Model file for the job. Use its own axes, mm. A direction names the side the tool comes from. Round coordinates to 2 decimals unless told otherwise and drop trailing zeros. Order: outer loops, then holes, each group sorted by start corner. A loop starts at its lowest first (then second) coordinate and runs counter-clockwise, first axis right, second up. Notation, with made-up numbers: (8, 24) - (64, 24) arc R25 ccw to (64, 43) - close; hole circle Ø4 at (54, -36.5). An arc over 180 degrees is marked (long way). Write item = value, one per line.
```python
from build123d import *

# Parameters (mm, degrees)
R_VOL_MINCE1_OUTLINE_W = 0.5
R_VOL_MINCE1_OUTLINE_H = 1
CONG_2_R               = 8
CONG_3_R               = 8


# Read off the part's stored shape, not the designer's step: Révol.-Mince1
with BuildPart() as part:
    # Révol.-Mince1 outline → Révol.-Mince1 (revolve)
    with BuildSketch(Plane.XY):
        Polygon((2.5, 5), (2.5, 0), (7, 0), (7, 23.528490035), (26.111064682, 23.528490035), (29, 0), (34.646665968, 0), (34.646665968, 3), (30.646665968, 3), (27.880515211, 25.528490035), (5, 25.528490035), (5, 5), align=None)
        with Locations((4.75, 2.5)):
            Rectangle(R_VOL_MINCE1_OUTLINE_W, R_VOL_MINCE1_OUTLINE_H, mode=Mode.SUBTRACT)
    revolve(axis=Axis((0, 0, 0), (0, 1, 0)))

    # Congé2
    cong_2_edges = [part.edges().sort_by_distance(p)[0] for p in [
        (-26.111064682, 23.528490035, 0),
    ]]
    fillet(cong_2_edges, radius=CONG_2_R)

    # Congé3
    cong_3_edges = [part.edges().sort_by_distance(p)[0] for p in [
        (-7, 23.528490035, 0),
    ]]
    fillet(cong_3_edges, radius=CONG_3_R)


solid = part.part
```
1) Wall check: line 1 along Z through (x, y) = (-0.5, 4.75); line 2 along Z through (x, y) = (0, 16); line 3 along X through (y, z) = (4.05, 0). Give the ranges that are in metal, low to high.
Conclusion:
line_1 = -30.43 to -28.41, -6.98 to -2.45, 2.45 to 6.98, 28.41 to 30.43
line_2 = -29.05 to -27.04, -7.01 to -5, 5 to 7.01, 27.04 to 29.05
line_3 = -30.52 to -28.5, -7 to -2.5, 2.5 to 7, 28.5 to 30.52
2) Mould opens along Z. For faces 6 (the face through (7.9, 0, 28.1)), 7 (the face through (6.466, 7.873, 2.681)), 8 (the face through (-6.27, 16.93, 28.25)) say: +Z half, -Z half, draft (parallel to the pull), parting line (faces both ways), or undercut.
Conclusion:
face_6 = draft
face_7 = undercut
face_8 = parting line
3) Cut at C-C (y = 18). Write the cut outline in (x, z), and give its area (3 significant figures).
Conclusion:
outline = circle Ø57.61 at (0, 0); circle Ø14.78 at (0, 0); hole circle Ø53.28 at (0, 0); hole circle Ø10 at (0, 0)
area = 470 mm^2
4) Cut at A-A (x = 0). Give the number of separate pieces and of enclosed holes in the cut face, and give its area (3 significant figures).
Conclusion:
separate_pieces = 2
enclosed_holes = 2
area = 376 mm^2
5) Flat gauge pins, fed straight in: pin 1 Ø5 at (x, z) = (-1, -2) entering from +Y; pin 2 Ø8 at (x, y) = (-21, 4) entering from +Z; pin 3 Ø2 at (y, z) = (21, -13) entering from -X. Where does each tip first touch, or does it go through?
Conclusion:
pin_1 = 5
pin_2 = 30.12
pin_3 = -25.8
6) 3-axis set-ups, long thin cutter, end or side, ignore diameter. For faces 1 (the face through (-0.59, 2.51, -4.46)), 2 (the face through (-1.08, 15.12, 4.88)), 3 (the face through (0, 0, 3)), 4 (the face through (32.005, 1.521, 13.27)), 5 (the face through (-14, 23.528, -6)): which of +Z, -Z, +X, -X, +Y, -Y reach the whole face in a straight line?
Conclusion:
face_1 = none
face_2 = +Y
face_3 = +Z, -Z, +X, -X, -Y
face_4 = +Y, -Y
face_5 = -Y
